```python
from build123d import *
from OCP.BRepAlgoAPI import BRepAlgoAPI_Cut
from OCP.TopTools import TopTools_ListOfShape

# Parameters (mm, degrees)
BOSS_EXTRUDE1_DEPTH = 11
SKETCH2_R           = 1
CUT_EXTRUDE1_DEPTH  = 49.17740653
SKETCH3_R           = 4
SKETCH3_R_2         = 1.25
SKETCH3_R_3         = 1
CUT_EXTRUDE3_DEPTH  = 56.793832843
BOSS_EXTRUDE2_DEPTH = 39.1
FILLET1_R           = 2
FILLET2_START       = -11
FILLET2_DEPTH       = 22.55
FILLET2_START_2     = -10.998352219
FILLET2_2_DEPTH     = 21.998352219
FILLET2_START_3     = -13
FILLET2_3_DEPTH     = 26
FILLET2_4_OUTLINE_W = 0.045411726
FILLET2_4_OUTLINE_H = 1
FILLET2_4_DEPTH     = 22


with BuildPart() as part:
    # Sketch1 → Boss-Extrude1 (new, symmetric)
    with BuildSketch(Plane.XY):
        Polygon((-16.25, 0), (16.25, 0), (16.25, 44), (-16.25, 44), (-16.25, 42.55), (14.8, 42.55), (14.8, 1.45), (-16.25, 1.45), align=None)
    extrude(amount=BOSS_EXTRUDE1_DEPTH, both=True)

    # Sketch2 → Cut-Extrude1 (cut, through all)
    with BuildSketch(Plane(origin=(0, 44, 0), x_dir=(1, 0, 0), z_dir=(0, 1, 0))):
        with BuildLine():
            Line((14.754588274, -11.001647781), (-14.245411726, -11.001647781))
            ThreePointArc((-14.245411726, -11.001647781), (-14.286004596, -11.001235793), (-14.326580741, -11))
            Line((-14.326580741, -11), (-16.25, -11))
            Line((-16.25, -11), (-16.25, 11))
            Line((-16.25, 11), (14.754588274, 11))
            Line((14.754588274, 11), (14.754588274, 13.363467794))
            Line((14.754588274, 13.363467794), (-19.651643458, 13.363467794))
            Line((-19.651643458, 13.363467794), (-19.651643458, -13.173756318))
            Line((-19.651643458, -13.173756318), (14.754588274, -13.173756318))
            Line((14.754588274, -13.173756318), (14.754588274, -11.001647781))
        make_face()
        with Locations(Location((-13.745411726, -8.001647781, 0), (0, 0, 180))):
            Circle(SKETCH2_R)
        with Locations(Location((-8.088557477, -5.658502031, 0), (0, 0, 180))):
            Circle(SKETCH2_R)
        with BuildLine():
            Line((1.254588274, 4.998352219), (-0.745411726, 4.998352219))
            ThreePointArc((-0.745411726, 4.998352219), (-1.452518507, 4.705459), (-1.745411726, 3.998352219))
            Line((-1.745411726, 3.998352219), (-1.745411726, -4.001647781))
            ThreePointArc((-1.745411726, -4.001647781), (-1.452518507, -4.708754562), (-0.745411726, -5.001647781))
            Line((-0.745411726, -5.001647781), (1.254588274, -5.001647781))
            ThreePointArc((1.254588274, -5.001647781), (1.961695055, -4.708754562), (2.254588274, -4.001647781))
            Line((2.254588274, -4.001647781), (2.254588274, 3.998352219))
            ThreePointArc((2.254588274, 3.998352219), (1.961695055, 4.705459), (1.254588274, 4.998352219))
        make_face()
        with BuildLine():
            Line((6.254588274, 3.998352219), (6.254588274, -4.001647781))
            ThreePointArc((6.254588274, -4.001647781), (6.547481493, -4.708754562), (7.254588274, -5.001647781))
            Line((7.254588274, -5.001647781), (9.254588274, -5.001647781))
            ThreePointArc((9.254588274, -5.001647781), (9.961695055, -4.708754562), (10.254588274, -4.001647781))
            Line((10.254588274, -4.001647781), (10.254588274, 3.998352219))
            ThreePointArc((10.254588274, 3.998352219), (9.961695055, 4.705459), (9.254588274, 4.998352219))
            Line((9.254588274, 4.998352219), (7.254588274, 4.998352219))
            ThreePointArc((7.254588274, 4.998352219), (6.547481493, 4.705459), (6.254588274, 3.998352219))
        make_face()
        with Locations(Location((4.254588274, -8.001647781, 0), (0, 0, 180))):
            Circle(SKETCH2_R)
        with Locations(Location((-5.745411726, -0.001647781, 0), (0, 0, 180))):
            Circle(SKETCH2_R)
        with Locations(Location((-8.088557477, 5.655206468, 0), (0, 0, 180))):
            Circle(SKETCH2_R)
        with Locations(Location((4.254588274, 7.998352219, 0), (0, 0, 180))):
            Circle(SKETCH2_R)
        with Locations(Location((-13.745411726, 7.998352219, 0), (0, 0, 180))):
            Circle(SKETCH2_R)
        with BuildLine():
            Line((-16.25, -11), (-14.326580741, -11))
            ThreePointArc((-14.326580741, -11), (-15.688037463, -10.386866531), (-16.245411726, -9.001647781))
            Line((-16.245411726, -9.001647781), (-16.245411726, -6.001647781))
            ThreePointArc((-16.245411726, -6.001647781), (-15.659625289, -4.587434219), (-14.245411726, -4.001647781))
            Line((-14.245411726, -4.001647781), (-13.745411726, -4.001647781))
            ThreePointArc((-13.745411726, -4.001647781), (-9.745411726, -0.001647781), (-13.745411726, 3.998352219))
            Line((-13.745411726, 3.998352219), (-14.245411726, 3.998352219))
            ThreePointArc((-14.245411726, 3.998352219), (-15.659625289, 4.584138657), (-16.245411726, 5.998352219))
            Line((-16.245411726, 5.998352219), (-16.245411726, 8.998352219))
            ThreePointArc((-16.245411726, 8.998352219), (-15.659625289, 10.412565781), (-14.245411726, 10.998352219))
            Line((-14.245411726, 10.998352219), (14.754588274, 10.998352219))
            Line((14.754588274, 10.998352219), (14.754588274, 11))
            Line((14.754588274, 11), (-16.25, 11))
            Line((-16.25, 11), (-16.25, -11))
        make_face()
    extrude(amount=-CUT_EXTRUDE1_DEPTH, mode=Mode.SUBTRACT)

    # Sketch3 → Cut-Extrude3 (cut, through all)
    with BuildSketch(Plane(origin=(16.25, 0, 0), x_dir=(0, 0, -1), z_dir=(1, 0, 0))):
        with Locations((0, 22.05)):
            Circle(SKETCH3_R)
        with BuildLine():
            Line((3, 38.05), (-3, 38.05))
            ThreePointArc((-3, 38.05), (-3.707106781, 37.757106781), (-4, 37.05))
            Line((-4, 37.05), (-4, 34.55))
            ThreePointArc((-4, 34.55), (-3.707106781, 33.842893219), (-3, 33.55))
            Line((-3, 33.55), (3, 33.55))
            ThreePointArc((3, 33.55), (3.707106781, 33.842893219), (4, 34.55))
            Line((4, 34.55), (4, 37.05))
            ThreePointArc((4, 37.05), (3.707106781, 37.757106781), (3, 38.05))
        make_face()
        with Locations((3.307494509, 30.05621399)):
            Circle(SKETCH3_R_2)
        with Locations((8, 30.05)):
            Circle(SKETCH3_R_2)
        with Locations((5.656854249, 27.706854249)):
            Circle(SKETCH3_R_3)
        with Locations((8, 25.372496408)):
            Circle(SKETCH3_R_2)
        with Locations((8, 22.05)):
            Circle(SKETCH3_R_3)
        with Locations((0, 30.05)):
            Circle(SKETCH3_R_3)
        with Locations((-3.322496408, 30.05)):
            Circle(SKETCH3_R_2)
        with Locations((-8, 30.05)):
            Circle(SKETCH3_R_2)
        with Locations((-5.656854249, 27.706854249)):
            Circle(SKETCH3_R_3)
        with Locations((-8.00621399, 25.357494509)):
            Circle(SKETCH3_R_2)
        with Locations((-8, 22.05)):
            Circle(SKETCH3_R_3)
        with BuildLine():
            Line((3, 10.55), (-3, 10.55))
            ThreePointArc((-3, 10.55), (-3.707106781, 10.257106781), (-4, 9.55))
            Line((-4, 9.55), (-4, 7.05))
            ThreePointArc((-4, 7.05), (-3.707106781, 6.342893219), (-3, 6.05))
            Line((-3, 6.05), (3, 6.05))
            ThreePointArc((3, 6.05), (3.707106781, 6.342893219), (4, 7.05))
            Line((4, 7.05), (4, 9.55))
            ThreePointArc((4, 9.55), (3.707106781, 10.257106781), (3, 10.55))
        make_face()
        with Locations((-8, 4.55)):
            Circle(SKETCH3_R_2)
        with Locations((8, 4.55)):
            Circle(SKETCH3_R_2)
        with Locations((8, 14.05)):
            Circle(SKETCH3_R_2)
        with Locations((8.00621399, 18.742505491)):
            Circle(SKETCH3_R_2)
        with Locations((5.656854249, 16.393145751)):
            Circle(SKETCH3_R_3)
        with Locations((3.322496408, 14.05)):
            Circle(SKETCH3_R_2)
        with Locations((0, 14.05)):
            Circle(SKETCH3_R_3)
        with Locations((-3.307494509, 14.04378601)):
            Circle(SKETCH3_R_2)
        with Locations((-8, 18.727503592)):
            Circle(SKETCH3_R_2)
        with Locations((-8, 14.05)):
            Circle(SKETCH3_R_2)
        with Locations((8, 39.55)):
            Circle(SKETCH3_R_2)
        with Locations((-8, 39.55)):
            Circle(SKETCH3_R_2)
        with Locations((-5.656854249, 16.393145751)):
            Circle(SKETCH3_R_3)
    extrude(amount=-CUT_EXTRUDE3_DEPTH, mode=Mode.SUBTRACT)

    # Sketch4 → Boss-Extrude2 (add)
    with BuildSketch(Plane(origin=(0, 2.45, 0), x_dir=(1, 0, 0), z_dir=(0, 1, 0))):
        with BuildLine():
            Line((16.25, -11), (16.25, -11.55))
            ThreePointArc((16.25, -11.55), (15.825304833, -12.575304833), (14.8, -13))
            Line((14.8, -13), (11.45, -13))
            Line((11.45, -13), (11.45, -11.55))
            Line((11.45, -11.55), (14.8, -11.55))
            Line((14.8, -11.55), (14.8, -11))
            Line((14.8, -11), (16.25, -11))
        make_face()
    boss_extrude2 = extrude(amount=BOSS_EXTRUDE2_DEPTH)

    # Mirror1: Boss-Extrude2 across plane
    add(boss_extrude2.mirror(Plane.XY))

    # Fillet1
    fillet1_edges = [part.edges().sort_by_distance(p)[0] for p in [
        (11.45, 2.45, 12.275),
        (11.45, 41.55, 12.275),
        (11.45, 2.45, -12.275),
        (11.45, 41.55, -12.275),
    ]]
    fillet(fillet1_edges, radius=FILLET1_R)


with BuildPart() as fillet2_tool:
    # Fillet2: read off the stored shape, not the designer's step
    # Fillet2 outline → Fillet2 (new body)
    with BuildSketch(Plane.XY.offset(FILLET2_START)):
        with BuildLine():
            ThreePointArc((14.754588253, 43.999992983), (15.812281126, 43.559036737), (16.25, 42.5))
            Line((16.25, 42.5), (16.25, 44))
            Line((16.25, 44), (14.754588253, 43.999992983))
        make_face()
        with BuildLine():
            ThreePointArc((16.25, 1.5), (15.812281126, 0.440963263), (14.754588253, 7.017e-06))
            Line((14.754588253, 7.017e-06), (16.25, 0))
            Line((16.25, 0), (16.25, 1.5))
        make_face()
    extrude(amount=FILLET2_DEPTH)


with BuildPart() as part_1:
    add(part.part)

    # Fillet2: cut by fillet2_tool, with a tolerance
    fillet2_stock = TopTools_ListOfShape()
    fillet2_stock.Append(part_1.part.wrapped)
    fillet2_tools = TopTools_ListOfShape()
    fillet2_tools.Append(fillet2_tool.part.wrapped)
    fillet2_cut = BRepAlgoAPI_Cut()
    fillet2_cut.SetArguments(fillet2_stock)
    fillet2_cut.SetTools(fillet2_tools)
    fillet2_cut.SetFuzzyValue(0.00001)
    fillet2_cut.Build()
    add(Compound.cast(fillet2_cut.Shape()).solids(), mode=Mode.REPLACE)


with BuildPart() as fillet2_2_tool:
    # Fillet2 2 outline → Fillet2 2 (new body)
    with BuildSketch(Plane.XY.offset(FILLET2_START_2)):
        with BuildLine():
            Line((13.3, 1.45), (14.8, 1.45))
            Line((14.8, 1.45), (14.8, 2.95))
            ThreePointArc((14.8, 2.95), (14.360660172, 1.889339828), (13.3, 1.45))
        make_face()
    extrude(amount=FILLET2_2_DEPTH)


with BuildPart() as part_2:
    add(part_1.part)


with BuildPart() as part_3:
    # Fillet2 2: joined with fillet2_2_tool
    add(part_2.part.fuse(fillet2_2_tool.part, tol=0.00001))


with BuildPart() as fillet2_3_tool:
    # Fillet2 3 outline → Fillet2 3 (new body)
    with BuildSketch(Plane.XY.offset(FILLET2_START_3)):
        with BuildLine():
            Line((14.714213563, 2.45), (14.8, 2.45))
            Line((14.8, 2.45), (14.8, 2.95))
            ThreePointArc((14.8, 2.95), (14.77839784, 2.696347032), (14.714213563, 2.45))
        make_face()
    extrude(amount=FILLET2_3_DEPTH)


with BuildPart() as part_4:
    add(part_3.part)


with BuildPart() as part_5:
    # Fillet2 3: joined with fillet2_3_tool
    add(part_4.part.fuse(fillet2_3_tool.part, tol=0.00001))


with BuildPart() as fillet2_4_tool:
    # Fillet2 4 outline → Fillet2 4 (new body)
    with BuildSketch(Plane.XY.offset(FILLET2_START)):
        with Locations((14.777294137, 1.95)):
            Rectangle(FILLET2_4_OUTLINE_W, FILLET2_4_OUTLINE_H)
    extrude(amount=FILLET2_4_DEPTH)


with BuildPart() as part_6:
    add(part_5.part)


with BuildPart() as part_7:
    # Fillet2 4: joined with fillet2_4_tool
    add(part_6.part.fuse(fillet2_4_tool.part, tol=0.00001))


solid = part_7.part
```
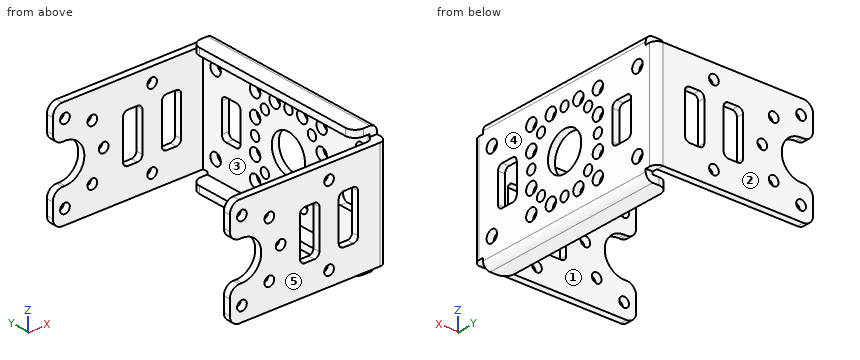
Read the model definition and answer for the solid it produces. Units are mm, in the model's axes. Face numbers are marked on the shaded views. A direction names the side the tool comes from. Give positions to 0.01 mm unless a question says otherwise; leave off trailing zeros. Write each loop counter-clockwise with the first axis right and the second up, starting at its lowest first coordinate (ties: lowest second). Pieces come first, ordered by that corner, then holes. Notation, with made-up numbers: M 83,-8 L 138,-8 A33 cw 138,25 Z; hole C 40.5,16 d4. An arc over 180 degrees is marked long. Put each result on its own line as item: value. Start each with the question number.
1. Which of the six approach directions +Z, -Z, +X, -X, +Y, -Y give full straight-line access (tool end or side, diameter ignored) to the marked faces 1 and 2?
2. Each of these flat-tipped pins is pushed along its axis until it touches: pin 1 Ø5 at (y, z) = (23, 1) entering from +X; pin 2 Ø1.6 at (x, z) = (15.5, 11.5) entering from -Y; pin 3 Ø1.2 at (x, y) = (-5.5, 1) entering from +Z; pin 4 Ø12 at (y, z) = (32, 10) entering from -X. Where does it stop, or does it pass through?
3. The part is cut by section A-A, the plane y = 22.05. Give the vertices of the cut face in (x, z).
4. The part is cut by section B-B, the plane x = -12. Give the vertices of the cut face in (y, z).
5. The part is cut by section D-D, the plane z = 7.5. Give the number of separate pieces and of enclosed holes in the cut face, and give its area (3 significant figures).
6. For a pull along Y with two mould halves and no side action, classify the marked faces 3, 4 and 5 as released by +Y, released by -Y, zero draft, split by the parting line, or undercut.
7. Consider line 1 along Y through (x, z) = (-8.5, 1.5); line 2 along Z through (x, y) = (13, 39); line 3 along X through (y, z) = (22.5, -10.5). Determine where each line is inside the solid, lowest interval first.
8. The part is cut by section C-C, the plane y = 36.5. Give the vertices of the cut face in (x, z), and give its area (3 significant figures).
Final values:
1. face 1: +Z, -Z, -X
1. face 2: +Z, -Z, +X, -X, +Y
2. pin 1: passes through
2. pin 2: stops at y = 0.01
2. pin 3: stops at z = 11
2. pin 4: stops at x = 11.45
3. outline: M 11.45,-13 L 14.8,-13 A1.45 ccw 16.25,-11.55 L 16.25,-9 L 14.8,-9 L 14.8,-11.55 L 11.45,-11.55 Z; M 11.45,11.55 L 14.8,11.55 L 14.8,9 L 16.25,9 L 16.25,11.55 A1.45 ccw 14.8,13 L 11.45,13 Z; M 14.8,-7 L 16.25,-7 L 16.25,-4 L 14.8,-4 Z; M 14.8,4 L 16.25,4 L 16.25,7 L 14.8,7 Z
4. outline: M 0,-11 L 1.45,-11 L 1.45,-3.6 L 0,-3.6 Z; M 0,3.6 L 1.45,3.6 L 1.45,11 L 0,11 Z; M 42.55,-11 L 44,-11 L 44,-3.6 L 42.55,-3.6 Z; M 42.55,3.6 L 44,3.6 L 44,11 L 42.55,11 Z
5. separate pieces: 12
5. enclosed holes: 0
5. area: 121 mm²
6. face 3: undercut
6. face 4: zero draft
6. face 5: released by -Y
7. line 1: y = 0 to 1.45, 42.55 to 44
7. line 2: z = -13 to -11.55, 11.55 to 13
7. line 3: x = 14.8 to 16.25
8. outline: M 11.45,-13 L 14.8,-13 A1.45 ccw 16.25,-11.55 L 16.25,-4 L 14.8,-4 L 14.8,-11.55 L 11.45,-11.55 Z; M 11.45,11.55 L 14.8,11.55 L 14.8,4 L 16.25,4 L 16.25,11.55 A1.45 ccw 14.8,13 L 11.45,13 Z
8. area: 34.9 mm²
